Geometry check sheet. Reference: the model listing, model coordinates, mm. Face numbers are marked on the shaded views. A direction names the side the tool comes from. Round coordinates to 2 decimals unless told otherwise and drop trailing zeros. Write each loop counter-clockwise with the first axis right and the second up, starting at its lowest first coordinate (ties: lowest second). Pieces come first, ordered by that corner, then holes.
Item 1: Cross-section at D-D (y = 2.25). Enter the section's corners in (x, z), then the cut area to 3 significant figures.
Item 2: Cross-section at A-A (y = 0.5). Enter the section's corners in (x, z), then the cut area to 3 significant figures.
Item 3: Draft check along Y on the marked faces 1, 2, 3 and 4. Enter one of: pulls with the +Y half, pulls with the -Y half, needs draft (parallel to the pull), parting line crosses it, or undercut.
Item 4: Depth check by flat-ended pin: P1, Ø4, axis at x = 0, y = 0, coming from the +Z side. Enter the tip coordinate at first touch or a pass-through.
Item 5: Access from +Z, -Z, +X, -X, +Y, -Y to the whole of each face (thin tool, end or side, straight path). Record for the marked faces 5 and 6.
Item 6: Cross-section at B-B (x = -25). Enter the section's corners in (y, z) (3 decimals), then the cut area to 3 significant figures.
Item 7: Cross-section at C-C (z = 0.6). State how many separate pieces and enclosed holes the cut face has, then the cut area to 3 significant figures.
Item 8: Scan lines: probe 1 along Y at (x, z) = (-16, 0.9); probe 2 along Y at (x, z) = (0, 1) (3 decimals). Record each from-to range of solid material in increasing order.
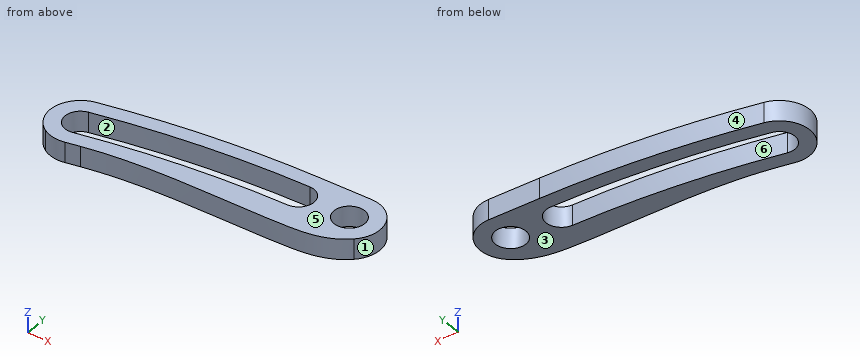
from build123d import *

# Parameters (mm, degrees)
SKETCH_2_R          = 1.515
EXTRUDE_2_DEPTH     = 2
EXTRUDE_START       = -2
EXTRUDE_3_OUTLINE_R = 1.515
EXTRUDE_3_DEPTH     = 2


with BuildPart() as part:
    # 草图2 → 凸台-拉伸2 (new body)
    with BuildSketch(Plane.XY):
        with BuildLine():
            Line((-4.501e-06, 3), (-4.996999856, 2.999992503))
            ThreePointArc((-4.996999856, 2.999992503), (-15.348887441, 2.488874451), (-25.596998621, 0.939992446))
            ThreePointArc((-25.596998621, 0.939992446), (-27.93999256, -2.596998062), (-24.403001606, -4.939991329))
            ThreePointArc((-24.403001606, -4.939991329), (-14.75186649, -3.481335038), (-5.003000142, -2.999990956))
            ThreePointArc((-5.003000143, -2.999991003), (-5.001500071, -2.999992128), (-5, -2.999994003))
            Line((-5, -2.999994003), (-3.598e-06, -3))
            ThreePointArc((-3.598e-06, -3), (3, 4.51e-07), (-4.501e-06, 3))
        make_face()
        Circle(SKETCH_2_R, mode=Mode.SUBTRACT)
        with BuildLine():
            ThreePointArc((-4.998474924, 1.524999237), (-3.475000763, -0.001525076), (-5.001525076, -1.524999237))
            ThreePointArc((-5.001525076, -1.524999237), (-14.898633731, -2.013662689), (-24.696525076, -3.494499237))
            ThreePointArc((-24.696525076, -3.494499237), (-26.494499237, -2.303474924), (-25.303474924, -0.505500763))
            ThreePointArc((-25.303474924, -0.505500763), (-15.202120074, 1.021200741), (-4.998474924, 1.524999237))
        make_face(mode=Mode.SUBTRACT)
    extrude(amount=EXTRUDE_2_DEPTH)

    # 凸台-拉伸3: read off the stored shape, not the designer's step
    # 凸台-拉伸3 outline → 凸台-拉伸3 (add)
    with BuildSketch(Plane.XY.offset(2).offset(EXTRUDE_START)):
        with BuildLine():
            ThreePointArc((-25.596998507, 0.939991888), (-27.939991888, -2.596998507), (-24.403001493, -4.939991888))
            ThreePointArc((-24.403001493, -4.939991888), (-23.740335049, -4.807830903), (-23.076763905, -4.680290004))
            add(Edge.make_bspline(
                [(2.0353099, -2.203976772), (0.364621675, -3.746809857), (-8.353685573, -4.252255019), (-16.667064883, -3.471457034), (-23.076763905, -4.680290004)],
                knots=[0, 0, 0, 0, 0.237995806, 1, 1, 1, 1], degree=3))
            ThreePointArc((2.0353099, -2.203976772), (2.79391492, 1.092721109), (-4.501e-06, 3))
            Line((-4.501e-06, 3), (-4.996999856, 2.999992413))
            ThreePointArc((-4.996999856, 2.999992413), (-15.348887454, 2.48887454), (-25.596998507, 0.939991888))
        make_face()
        with BuildLine():
            ThreePointArc((-24.696525076, -3.494499237), (-26.494499237, -2.303474924), (-25.303474924, -0.505500763))
            ThreePointArc((-25.303474924, -0.505500763), (-15.202120074, 1.021200741), (-4.998474924, 1.524999237))
            ThreePointArc((-4.998474924, 1.524999237), (-3.475000763, -0.001525076), (-5.001525076, -1.524999237))
            ThreePointArc((-5.001525076, -1.524999237), (-14.898633731, -2.013662689), (-24.696525076, -3.494499237))
        make_face(mode=Mode.SUBTRACT)
        Circle(EXTRUDE_3_OUTLINE_R, mode=Mode.SUBTRACT)
    extrude(amount=EXTRUDE_3_DEPTH)


solid = part.part
Resolved:
1. outline: (-17.51, 0) - (1.98, 0) - (1.98, 2) - (-17.51, 2) - close
1. area: 39.0 mm2
2. outline: (-26.66, 0) - (-19.49, 0) - (-19.49, 2) - (-26.66, 2) - close; (-3.56, 0) - (-1.43, 0) - (-1.43, 2) - (-3.56, 2) - close; (1.43, 0) - (2.96, 0) - (2.96, 2) - (1.43, 2) - close
2. area: 21.6 mm2
3. face 1: parting line crosses it
3. face 2: undercut
3. face 3: needs draft
3. face 4: pulls with the +Y half
4. P1: stops at z = 2
5. face 5: +Z, +X, -X, +Y, -Y
5. face 6: +Z, -Z
6. outline: (-5, 0) - (-3.525, 0) - (-3.525, 2) - (-5, 2) - close; (-0.444, 0) - (1.059, 0) - (1.059, 2) - (-0.444, 2) - close
6. area: 5.96 mm2
7. separate pieces: 1
7. enclosed holes: 2
7. area: 116 mm2
8. probe 1: y = -3.95 to -2.13, 0.94 to 2.42
8. probe 2: y = -3.413 to -1.515, 1.515 to 3
